from build123d import *

# Parameters (mm, degrees)
SKETCH1_W           = 27.94
SKETCH1_H           = 53.34
BOSS_EXTRUDE1_DEPTH = 9.74725
CUT_EXTRUDE1_DEPTH  = 27.94
FILLET1_R           = 5.334
FILLET2_R           = 5.334
SHELL1_T            = -2.54
SKETCH3_R           = 10.16
CUT_EXTRUDE2_DEPTH  = 24.13
SKETCH5_W           = 10.795
SKETCH5_H           = 1.5875
CUT_EXTRUDE3_DEPTH  = 2.54
BOSS_EXTRUDE2_DEPTH = 1.5875


with BuildPart() as part:
    # Sketch1 → Boss-Extrude1 (new, symmetric)
    with BuildSketch(Plane(origin=(0, 0, 0), x_dir=(1, 0, 0), z_dir=(0, 1, 0))):
        Rectangle(SKETCH1_W, SKETCH1_H)
    extrude(amount=BOSS_EXTRUDE1_DEPTH, both=True)

    # Sketch2 → Cut-Extrude1 (cut)
    with BuildSketch(Plane(origin=(13.97, 0, 0), x_dir=(0, 0, -1), z_dir=(1, 0, 0))):
        with BuildLine():
            Line((-26.67, 9.74725), (-26.67, 4.03225))
            Line((-26.67, 4.03225), (3.81, 4.03225))
            ThreePointArc((3.81, 4.03225), (8.850435754, 8.238878491), (15.24, 9.74725))
            Line((15.24, 9.74725), (-26.67, 9.74725))
        make_face()
        with BuildLine():
            Line((26.67, 9.74725), (15.24, 9.74725))
            ThreePointArc((15.24, 9.74725), (21.629564246, 8.238878491), (26.67, 4.03225))
            Line((26.67, 4.03225), (26.67, 9.74725))
        make_face()
    extrude(amount=-CUT_EXTRUDE1_DEPTH, mode=Mode.SUBTRACT)

    # Fillet1
    fillet1_edges = [part.edges().sort_by_distance(p)[0] for p in [
        (0, 4.03225, -3.81),
    ]]
    fillet(fillet1_edges, radius=FILLET1_R)

    # Fillet2
    fillet2_edges = [part.edges().sort_by_distance(p)[0] for p in [
        (0, 4.03225, -26.67),
    ]]
    fillet(fillet2_edges, radius=FILLET2_R)

    # Shell1
    shell1_openings = [part.faces().sort_by_distance(p)[0] for p in [
        (0, -9.74725, 0),
    ]]
    offset(amount=SHELL1_T, openings=shell1_openings, kind=Kind.INTERSECTION)

    # Sketch3 → Cut-Extrude2 (cut)
    with BuildSketch(Plane(origin=(0, 4.03225, 0), x_dir=(1, 0, 0), z_dir=(0, 1, 0))):
        with Locations(Location((0, -11.43, 0), (0, 0, 270))):
            Circle(SKETCH3_R)
    extrude(amount=-CUT_EXTRUDE2_DEPTH, mode=Mode.SUBTRACT)

    # Sketch5 → Cut-Extrude3 (cut)
    with BuildSketch(Plane(origin=(0, 0, -26.67), x_dir=(-1, 0, 0), z_dir=(0, 0, -1))):
        with Locations((0, -8.9535)):
            Rectangle(SKETCH5_W, SKETCH5_H)
    extrude(amount=-CUT_EXTRUDE3_DEPTH, mode=Mode.SUBTRACT)

    # Sketch4 → Boss-Extrude2 (add)
    with BuildSketch(Plane.XZ.offset(9.74725)):
        Polygon((-5.3975, -24.13), (-11.43, -24.13), (-11.43, 24.13), (11.43, 24.13), (11.43, -24.13), (5.3975, -24.13), (5.3975, -25.4), (12.7, -25.4), (12.7, 25.4), (-12.7, 25.4), (-12.7, -25.4), (-5.3975, -25.4), align=None)
    extrude(amount=BOSS_EXTRUDE2_DEPTH)


solid = part.part
Can you work these out from the model? Positions are in its coordinate system, mm. A direction names the side the tool comes from. Coordinates: 2 decimals unless noted, no trailing zeros. Write each loop counter-clockwise with the first axis right and the second up, starting at its lowest first coordinate (ties: lowest second). Pieces come first, ordered by that corner, then holes.
Q1. Imagine slicing it at C-C, the plane y = -1. List the corners of the cut face in (x, z) for me, plus the area to 3 significant figures.
Results found:
outline: (-13.97, -26.67) - (13.97, -26.67) - (13.97, 26.67) - (-13.97, 26.67) - close; hole (-11.43, -24.13) - (11.43, -24.13) - (11.43, 24.13) - (-11.43, 24.13) - close
area: 387 mm2
Q2. Imagine slicing it at B-B, the plane z = 11.43. List the corners of the cut face in (x, y) for me.
Results found:
outline: (-13.97, -9.75) - (-12.7, -9.75) - (-12.7, -11.33) - (-11.43, -11.33) - (-11.43, 1.49) - (-10.16, 1.49) - (-10.16, 4.03) - (-13.97, 4.03) - close; (10.16, 1.49) - (11.43, 1.49) - (11.43, -11.33) - (12.7, -11.33) - (12.7, -9.75) - (13.97, -9.75) - (13.97, 4.03) - (10.16, 4.03) - close
Q3. Which directions (+Z, -Z, +X, -X, +Y, -Y) give clear straight access to the entire face, cutting with the end or side of a thin tool? Please do faces 1 (the face through (-12.7, -11, 0)), 2 (the face through (-0.16, 2.07, -4.36)), 3 (the face through (12.7, -11, 0)), 4 (the face through (5.398, -9, -25)), 5 (the face through (9, -11, -25.4)).
Results found:
face 1: +Z, -Z, -X, -Y
face 2: -Y
face 3: +Z, -Z, +X, -Y
face 4: -Z, -Y
face 5: -Z, +X, -X, -Y
Q4. Please list where these lines run through material, in increasing order: L1, parallel to X at y = 2.7, z = 11.43; L2, parallel to X at y = -6, z = 9; L3, parallel to Z at x = 3.75, y = -6.75.
Results found:
L1: x = -13.97 to -10.16, 10.16 to 13.97
L2: x = -13.97 to -11.43, 11.43 to 13.97
L3: z = -26.67 to -24.13, 24.13 to 26.67
Q5. If we mould it in two halves opening along X, with no side actions, what happens to faces 6 (the face through (-5.398, -9, -25)), 7 (the face through (-0.2, 4.18, -26.21)), 8 (the face through (-13.97, -2, 0))? For each: +X half, -X half, draft (parallel to the pull), parting line (faces both ways), or undercut.
Results found:
face 6: undercut
face 7: draft
face 8: -X half
Q6. Imagine slicing it at A-A, the plane x = 0. List the corners of the cut face in (y, z) for me (1 decimal).
Results found:
outline: (-11.3, 24.1) - (1.5, 24.1) - (1.5, 21.6) - (4, 21.6) - (4, 26.7) - (-9.7, 26.7) - (-9.7, 25.4) - (-11.3, 25.4) - close; (-8.2, -26.7) - (2, -26.7) arc R5.3 ccw to (5.9, -25) arc R14.3 ccw to (5.6, -5.2) arc R5.3 cw to (4, -1.4) - (4, 1.3) - (1.5, 1.3) - (1.5, -1.4) arc R7.9 ccw to (3.8, -7) arc R11.7 cw to (4.1, -23.2) arc R2.8 cw to (2, -24.1) - (-8.2, -24.1) - close
Q7. Imagine slicing it at D-D, the plane z = -19.5. List the corners of the cut face in (x, y) for me, plus the area to 3 significant figures.
Results found:
outline: (-13.97, -9.75) - (-12.7, -9.75) - (-12.7, -11.33) - (-11.43, -11.33) - (-11.43, 6.41) - (11.43, 6.41) - (11.43, -11.33) - (12.7, -11.33) - (12.7, -9.75) - (13.97, -9.75) - (13.97, 9.1) - (-13.97, 9.1) - close
area: 161 mm2
Q8. For P1, Ø6, axis at x = 9.5, z = 9.5, coming from the +Y side; P2, Ø5, axis at x = 1.5, z = -9, coming from the +Y side; P3, Ø3, axis at x = -1.5, z = -25.5, coming from the -Y side; P4, Ø7, axis at x = 5.5, z = 11.5, coming from the -Y side, each with a flat end and sliding along its axis, tell me the tip position at first contact or that it passes through.
Results found:
P1: stops at y = 4.03
P2: stops at y = 9.25
P3: stops at y = -8.16
P4: passes through
